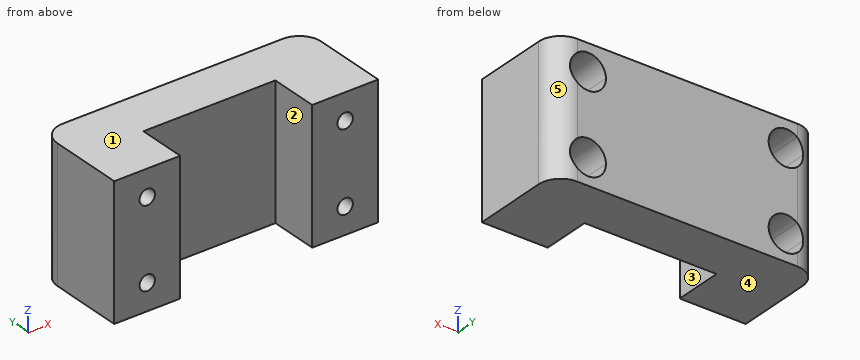
```python
from build123d import *

# Parameters (mm, degrees)
F1_DEPTH = 30
F2_R     = 1.75
F3_R     = 1.75
F4_DEPTH = 22.001
F5_R     = 1.75
F6_DEPTH = 10


with BuildPart() as f1:
    # F0 (on Top) → F1 (new body)
    with BuildSketch(Plane.XY):
        with BuildLine():
            Line((25, 22), (-25, 22))
            ThreePointArc((-25, 22), (-28.5355339059, 20.5355339059), (-30, 17))
            Line((-30, 17), (-30, 0))
            Line((-30, 0), (-15, 0))
            Line((-15, 0), (-15, 11))
            Line((-15, 11), (15, 11))
            Line((15, 11), (15, 0))
            Line((15, 0), (30, 0))
            Line((30, 0), (30, 17))
            ThreePointArc((30, 17), (28.5355339059, 20.5355339059), (25, 22))
        make_face()
    extrude(amount=F1_DEPTH)

    # F2 (on face) + F3 (on face) → F4 (cut, through all)
    with BuildSketch(Plane.XZ):
        with Locations((-22.5, 24)):
            Circle(F2_R)
        with Locations((-22.5, 6)):
            Circle(F2_R)
    with BuildSketch(Plane.XZ):
        with Locations((22.5, 6)):
            Circle(F3_R)
        with Locations((22.5, 24)):
            Circle(F3_R)
    extrude(amount=-F4_DEPTH, mode=Mode.SUBTRACT)

    # F5 (on face) → F6 (cut)
    with BuildSketch(Plane(origin=(0, 22, 0), x_dir=(-1, 0, 0), z_dir=(0, 1, 0))):
        with BuildLine():
            ThreePointArc((25, 20.8775010008), (26.1055512755, 22.2679491924), (26.5, 24))
            ThreePointArc((26.5, 24), (26.1055512755, 25.7320508076), (25, 27.1224989992))
            Line((25, 27.1224989992), (25, 20.8775010008))
        make_face()
        with BuildLine():
            Line((25, 20.8775010008), (25, 27.1224989992))
            ThreePointArc((25, 27.1224989992), (18.5, 24), (25, 20.8775010008))
        make_face()
        with Locations((22.5, 24)):
            Circle(F5_R, mode=Mode.SUBTRACT)
        with BuildLine():
            Line((25, 2.8775010008), (25, 9.1224989992))
            ThreePointArc((25, 9.1224989992), (18.5, 6), (25, 2.8775010008))
        make_face()
        with Locations((22.5, 6)):
            Circle(F5_R, mode=Mode.SUBTRACT)
        with BuildLine():
            ThreePointArc((26.5, 6), (26.1055512755, 7.7320508076), (25, 9.1224989992))
            Line((25, 9.1224989992), (25, 2.8775010008))
            ThreePointArc((25, 2.8775010008), (26.1055512755, 4.2679491924), (26.5, 6))
        make_face()
        with BuildLine():
            ThreePointArc((-18.5, 6), (-20.7679491924, 9.6055512755), (-25, 9.1224989992))
            Line((-25, 9.1224989992), (-25, 2.8775010008))
            ThreePointArc((-25, 2.8775010008), (-20.7679491924, 2.3944487245), (-18.5, 6))
        make_face()
        with Locations((-22.5, 6)):
            Circle(F5_R, mode=Mode.SUBTRACT)
        with BuildLine():
            Line((-25, 2.8775010008), (-25, 9.1224989992))
            ThreePointArc((-25, 9.1224989992), (-26.5, 6), (-25, 2.8775010008))
        make_face()
        with BuildLine():
            ThreePointArc((-18.5, 24), (-20.7679491924, 27.6055512755), (-25, 27.1224989992))
            Line((-25, 27.1224989992), (-25, 20.8775010008))
            ThreePointArc((-25, 20.8775010008), (-20.7679491924, 20.3944487245), (-18.5, 24))
        make_face()
        with Locations((-22.5, 24)):
            Circle(F5_R, mode=Mode.SUBTRACT)
        with BuildLine():
            Line((-25, 20.8775010008), (-25, 27.1224989992))
            ThreePointArc((-25, 27.1224989992), (-26.5, 24), (-25, 20.8775010008))
        make_face()
    extrude(amount=-F6_DEPTH, mode=Mode.SUBTRACT)


solid = f1.part
```
Source: CAD feature listing. Evaluate the final solid. Frame: model axes, mm. Face numbers are marked on the shaded views. A direction names the side the tool comes from. Give positions to 0.01 mm unless a question says otherwise; leave off trailing zeros. Write each loop counter-clockwise with the first axis right and the second up, starting at its lowest first coordinate (ties: lowest second). Pieces come first, ordered by that corner, then holes. Notation, with made-up numbers: (-9.5, -17.75) - (41.5, -17.75) arc R16 cw to (41.5, 12.25) - close; hole circle Ø11 at (-12, 62.5). An arc over 180 degrees is marked (long way). One line per item, written item: value. Start each with the question number.
Q1. First-contact query: pin 1 Ø4 at (x, z) = (22, 6.5) entering from +Y; pin 2 Ø9 at (x, z) = (-3, 21.5) entering from -Y. Flat tips, straight axial feed; report the tip coordinate or a pass-through.
Q2. Draft query along X for the marked faces 3, 4 and 5. Return one class per face: +X half, -X half, draft (parallel to the pull), parting line (faces both ways), or undercut.
Q3. Material intervals for probe 1 along Z at (x, y) = (-22.5, 4.5); probe 2 along X at (y, z) = (17.25, 6); probe 3 along X at (y, z) = (18.5, 26), sorted ascending. Write a range as from..to.
Q4. Set-up query: the marked faces 1 and 2. Return all of +Z, -Z, +X, -X, +Y, -Y with unobstructed straight access to the full face (end or side cutting, diameter ignored); none if empty.
Q5. Section query A-A, the plane x = 22.5. Return the cut outline in (y, z), then the cut area to 3 significant figures.
Q6. Section query C-C, the plane z = 17. Return the cut outline in (x, y), then the cut area to 3 significant figures.
Q7. Section query D-D, the plane y = 15. Return the cut outline in (x, z).
Q8. Section query B-B, the plane y = 5.5. Return the cut outline in (x, z).
Answer:
1. pin 1: stops at y = 12
1. pin 2: stops at y = 11
2. face 3: undercut
2. face 4: draft
2. face 5: +X half
3. probe 1: z = 0..4.25, 7.75..22.25, 25.75..30
3. probe 2: x = -29.99..-26.5, -18.5..18.5, 26.5..29.99
3. probe 3: x = -29.77..-25.96, -19.04..19.04, 25.96..29.77
4. face 1: +Z, +X, -X, +Y, -Y
4. face 2: +Z, -Z, -Y
5. outline: (0, 0) - (22, 0) - (22, 2) - (12, 2) - (12, 4.25) - (0, 4.25) - close; (0, 7.75) - (12, 7.75) - (12, 10) - (22, 10) - (22, 20) - (12, 20) - (12, 22.25) - (0, 22.25) - close; (0, 25.75) - (12, 25.75) - (12, 28) - (22, 28) - (22, 30) - (0, 30) - close
5. area: 416 mm2
6. outline: (-30, 0) - (-15, 0) - (-15, 11) - (15, 11) - (15, 0) - (30, 0) - (30, 17) arc R5 ccw to (25, 22) - (-25, 22) arc R5 ccw to (-30, 17) - close
6. area: 979 mm2
7. outline: (-30, 0) - (30, 0) - (30, 30) - (-30, 30) - close; hole circle Ø8 at (-22.5, 6); hole circle Ø8 at (-22.5, 24); hole circle Ø8 at (22.5, 6); hole circle Ø8 at (22.5, 24)
8. outline: (-30, 0) - (-15, 0) - (-15, 30) - (-30, 30) - close; (15, 0) - (30, 0) - (30, 30) - (15, 30) - close; hole circle Ø3.5 at (-22.5, 6); hole circle Ø3.5 at (-22.5, 24); hole circle Ø3.5 at (22.5, 6); hole circle Ø3.5 at (22.5, 24)
